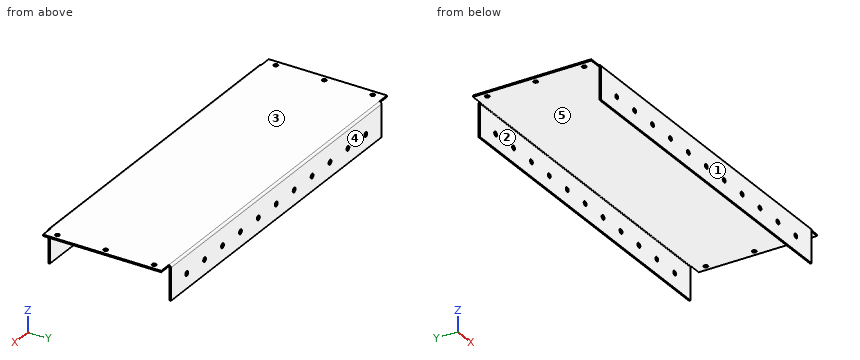
```python
from build123d import *

# Parameters (mm, degrees)
MODEL_W                        = 252.1
MODEL_H                        = 84
MODEL_R                        = 1.5
BASE_FLANGE1_DEPTH             = 1
EDGE_FLANGE1_STRIP_W           = 5
EDGE_FLANGE1_STRIP_H           = 1
EDGE_FLANGE1_STRIP_CUT_DEPTH   = 252.1
EDGE_FLANGE1_STRIP_2_W         = 5
EDGE_FLANGE1_STRIP_2_H         = 1
EDGE_FLANGE1_STRIP_CUT_2_DEPTH = 252.1
EDGE_FLANGE1_DEPTH             = 252.1
EDGE_FLANGE1_BEND_DEPTH        = 252.1
SKETCH13_R                     = 1.6
CUT_EXTRUDE1_DEPTH             = 155.468775162
SKETCH14_W                     = 8.4
SKETCH14_H                     = 24
CUT_EXTRUDE2_DEPTH             = 1.5


# Sheet-metal steps are written as plain solids
with BuildPart() as part:
    # Model → Base-Flange1 (new body)
    with BuildSketch(Plane.XY):
        Rectangle(MODEL_W, MODEL_H)
        with Locations((-122.05, 34)):
            Circle(MODEL_R, mode=Mode.SUBTRACT)
        with Locations((-122.05, -34)):
            Circle(MODEL_R, mode=Mode.SUBTRACT)
        with Locations((122.05, -34)):
            Circle(MODEL_R, mode=Mode.SUBTRACT)
        with Locations((122.05, 34)):
            Circle(MODEL_R, mode=Mode.SUBTRACT)
        with Locations((122.05, 0)):
            Circle(MODEL_R, mode=Mode.SUBTRACT)
        with Locations((-122.05, 0)):
            Circle(MODEL_R, mode=Mode.SUBTRACT)
    extrude(amount=-BASE_FLANGE1_DEPTH)

    # Edge-Flange1 strip (across the edge) → Edge-Flange1 strip cut (cut)
    with BuildSketch(Plane(origin=(126.05, -42, -1), x_dir=(0, 1, 0), z_dir=(-1, 0, 0))):
        with Locations((-2, -0.5)):
            Rectangle(EDGE_FLANGE1_STRIP_W, EDGE_FLANGE1_STRIP_H)
    extrude(amount=EDGE_FLANGE1_STRIP_CUT_DEPTH, mode=Mode.SUBTRACT)

    # Edge-Flange1 strip 2 (across the edge) → Edge-Flange1 strip cut 2 (cut)
    with BuildSketch(Plane(origin=(-126.05, 42, -1), x_dir=(0, -1, 0), z_dir=(1, 0, 0))):
        with Locations((-2, -0.5)):
            Rectangle(EDGE_FLANGE1_STRIP_2_W, EDGE_FLANGE1_STRIP_2_H)
    extrude(amount=EDGE_FLANGE1_STRIP_CUT_2_DEPTH, mode=Mode.SUBTRACT)

    # Edge-Flange1 section (across the edge) → Edge-Flange1 (add)
    with BuildSketch(Plane(origin=(126.05, -42, -1), x_dir=(0, 1, 0), z_dir=(-1, 0, 0))):
        with BuildLine():
            Line((-1, 0.5), (-1, 23))
            Line((-1, 23), (0, 23))
            Line((0, 23), (0, 0.5))
            ThreePointArc((0, 0.5), (0.146446609, 0.146446609), (0.5, 0))
            Line((0.5, 0), (0.5, -1))
            ThreePointArc((0.5, -1), (-0.560660172, -0.560660172), (-1, 0.5))
        make_face()
    extrude(amount=EDGE_FLANGE1_DEPTH)

    # Edge-Flange1 section 2 (across the edge) → Edge-Flange1 bend (add)
    with BuildSketch(Plane(origin=(-126.05, 42, -1), x_dir=(0, -1, 0), z_dir=(1, 0, 0))):
        with BuildLine():
            Line((-1, 0.5), (-1, 23))
            Line((-1, 23), (0, 23))
            Line((0, 23), (0, 0.5))
            ThreePointArc((0, 0.5), (0.146446609, 0.146446609), (0.5, 0))
            Line((0.5, 0), (0.5, -1))
            ThreePointArc((0.5, -1), (-0.560660172, -0.560660172), (-1, 0.5))
        make_face()
    extrude(amount=EDGE_FLANGE1_BEND_DEPTH)

    # Sketch13 → Cut-Extrude1 (cut, through all)
    with BuildSketch(Plane(origin=(0, 43, 0), x_dir=(1, 0, 0), z_dir=(0, 1, 0))):
        with Locations(Location((-100, 13.75, 0), (0, 0, 270))):
            Circle(SKETCH13_R)
        with Locations(Location((-80, 13.75, 0), (0, 0, 270))):
            Circle(SKETCH13_R)
        with Locations(Location((-60, 13.75, 0), (0, 0, 270))):
            Circle(SKETCH13_R)
        with Locations(Location((-40, 13.75, 0), (0, 0, 270))):
            Circle(SKETCH13_R)
        with Locations(Location((-20, 13.75, 0), (0, 0, 270))):
            Circle(SKETCH13_R)
        with Locations(Location((0, 13.75, 0), (0, 0, 270))):
            Circle(SKETCH13_R)
        with Locations(Location((20, 13.75, 0), (0, 0, 270))):
            Circle(SKETCH13_R)
        with Locations(Location((40, 13.75, 0), (0, 0, 270))):
            Circle(SKETCH13_R)
        with Locations(Location((60, 13.75, 0), (0, 0, 270))):
            Circle(SKETCH13_R)
        with Locations(Location((80, 13.75, 0), (0, 0, 270))):
            Circle(SKETCH13_R)
        with Locations(Location((100, 13.75, 0), (0, 0, 270))):
            Circle(SKETCH13_R)
    extrude(amount=-CUT_EXTRUDE1_DEPTH, mode=Mode.SUBTRACT)

    # Sketch14 → Cut-Extrude2 (cut)
    with BuildSketch(Plane(origin=(0, 43, 0), x_dir=(1, 0, 0), z_dir=(0, 1, 0))):
        with Locations((-121.85, 12)):
            Rectangle(SKETCH14_W, SKETCH14_H)
        with Locations((121.85, 12)):
            Rectangle(SKETCH14_W, SKETCH14_H)
    cut_extrude2 = extrude(amount=-CUT_EXTRUDE2_DEPTH, mode=Mode.SUBTRACT)

    # Mirror1: Cut-Extrude2 across plane
    add(cut_extrude2.mirror(Plane.ZX), mode=Mode.SUBTRACT)


solid = part.part
```
Here's how the part is built. I have some questions about the finished solid (model axes, mm). Face numbers are marked on the shaded views. A direction names the side the tool comes from. Give positions to 0.01 mm unless a question says otherwise; leave off trailing zeros. Loops run counter-clockwise (first coordinate to the right, second up) from the corner with the lowest first, then second, coordinate; pieces in that order, holes last. Notation, with made-up numbers: M -17.75,-8.75 L -3.75,-8.75 A14 cw -3.75,16.25 Z; hole C 22.25,-9.75 d9. An arc over 180 degrees is marked long. Return JSON: item names as keys, results as strings.
Item 1: Imagine slicing it at B-B on x = -76. List the corners of the cut face in (y, z) for me.
A:
{"outline": "M -43,-24 L -42,-24 L -42,-1.5 A0.5 cw -41.5,-1 L 41.5,-1 A0.5 cw 42,-1.5 L 42,-24 L 43,-24 L 43,-1.5 A1.5 ccw 41.5,0 L -41.5,0 A1.5 ccw -43,-1.5 Z"}
Item 2: Imagine slicing it at C-C on y = 19.5. List the corners of the cut face in (x, z) for me, then the cut area to 3 significant figures.
A:
{"outline": "M -126.05,-1 L 126.05,-1 L 126.05,0 L -126.05,0 Z", "area": "252 mm^2"}
Item 3: On a 3-axis mill with a long thin cutter (end or side, diameter ignored), from which of +Z, -Z, +X, -X, +Y, -Y can I reach the whole of each face in a straight line? I mean the marked faces 4 and 5. Say none if no direction works.
A:
{"face 4": "+Z, -Z, +X, -X, +Y", "face 5": "-Z, +X, -X"}
Item 4: I'm going to push flat-ended pins straight in: pin 1 Ø8 at (x, y) = (-56, 8) entering from -Z; pin 2 Ø0.8 at (y, z) = (-42, -15) entering from -X. Where does each tip first touch, or does it pass through?
A:
{"pin 1": "stops at z = -1", "pin 2": "stops at x = -117.65"}
Item 5: Imagine slicing it at A-A on z = -6.75. List the corners of the cut face in (x, y) for me, then the cut area to 3 significant figures.
A:
{"outline": "M -117.65,-43 L 117.65,-43 L 117.65,-42 L -117.65,-42 Z; M -117.65,42 L 117.65,42 L 117.65,43 L -117.65,43 Z", "area": "471 mm^2"}
Item 6: Please list where these lines run through material, in increasing order: line 1 (Y direction, x = 21.5, z = -10.75); line 2 (Z direction, x = 69, y = -21).
A:
{"line 1": "y = -43 to -42, 42 to 43", "line 2": "z = -1 to 0"}
Item 7: Thinking about a two-plate mould opening in Y: for the marked faces 1, 2 and 3, which applies, released by +Y, released by -Y, zero draft, split by the parting line, or undercut?
A:
{"face 1": "released by -Y", "face 2": "undercut", "face 3": "zero draft"}
